from build123d import *

# Parameters (mm, degrees)
SKETCH1_W           = 71.12
SKETCH1_H           = 71.12
BOSS_EXTRUDE1_DEPTH = 2.54
SKETCH2_R           = 15.24
CUT_EXTRUDE1_DEPTH  = 15.748


with BuildPart() as part:
    # Sketch1 → Boss-Extrude1 (new body)
    with BuildSketch(Plane(origin=(0, 0, 0), x_dir=(1, 0, 0), z_dir=(0, 1, 0))):
        with Locations((10.146850495, 4.656355231)):
            Rectangle(SKETCH1_W, SKETCH1_H)
    extrude(amount=-BOSS_EXTRUDE1_DEPTH)

    # Sketch2 → Cut-Extrude1 (cut)
    with BuildSketch(Plane(origin=(0, 0, 0), x_dir=(1, 0, 0), z_dir=(0, 1, 0))):
        with Locations(Location((10.146850495, 23.706355231, 0), (0, 0, 270))):
            Circle(SKETCH2_R)
    extrude(amount=-CUT_EXTRUDE1_DEPTH, mode=Mode.SUBTRACT)


solid = part.part
The model under review builds one solid part; all positions refer to its coordinate system, in mm. Give positions to 0.01 mm unless a question says otherwise; leave off trailing zeros. Order: outer loops, then holes, each group sorted by start corner. A loop starts at its lowest first (then second) coordinate and runs counter-clockwise, first axis right, second up. Notation, with made-up numbers: M 32,58.25 L 68,58.25 A5 cw 68,66.25 Z; hole C -23.5,9.25 d8. An arc over 180 degrees is marked long. One line per question, with ' | ' between items. Start each with the question number.
1) Consider section A-A, the plane x = 9. Give the boundary of the cut face in (y, z), then the cut area to 3 significant figures.
2) Clearance check with a flat-ended pin moving along its axis: P1, Ø8, axis at x = -10.5, z = 14.5, coming from the +Y side. State where the tip first meets the part, or that it passes through.
3) Mouldability with a two-part tool opening along X and no side actions: class faces 1 (the face through (10, -2.54, -5)), 2 (the face through (45.707, -1, -4)), 3 (the face through (0.87, -1.25, -35.8)) as pulls with the +X half, pulls with the -X half, needs draft (parallel to the pull), parting line crosses it, or undercut.
4) Wall thickness on L1, parallel to X at y = -1.75, z = -10; L2, parallel to Z at x = 5.5, y = -0.55; L3, parallel to Z at x = -2.5, y = -1.35: over which ranges is each line inside the solid? List them lowest first. Write a range as from..to.
5) Consider section C-C, the plane y = -1.9. Give the boundary of the cut face in (x, z), then the cut area to 3 significant figures.
6) Consider section B-B, the plane z = -19.5. Give the boundary of the cut face in (x, y), then the cut area to 3 significant figures.
Found:
1) outline: M -2.54,-40.22 L 0,-40.22 L 0,-38.9 L -2.54,-38.9 Z; M -2.54,-8.51 L 0,-8.51 L 0,30.9 L -2.54,30.9 Z | area: 103 mm²
2) P1: stops at y = 0
3) face 1: needs draft | face 2: pulls with the +X half | face 3: undercut
4) L1: x = -25.41..3.48, 16.81..45.71 | L2: z = -40.22..-38.22, -9.19..30.9 | L3: z = -40.22..-32.21, -15.2..30.9
5) outline: M -25.41,-40.22 L 45.71,-40.22 L 45.71,30.9 L -25.41,30.9 Z; hole C 10.15,-23.71 d30.48 | area: 4,330 mm²
6) outline: M -25.41,-2.54 L -4.5,-2.54 L -4.5,0 L -25.41,0 Z; M 24.79,-2.54 L 45.71,-2.54 L 45.71,0 L 24.79,0 Z | area: 106 mm²
